from build123d import *

# Parameters (mm, degrees)
BOX002_W          = 50
BOX002_H          = 10
BOX002_DEPTH      = 3
CYLINDER001_R     = 3
CYLINDER001_DEPTH = 5
CYLINDER_R        = 10
CYLINDER_DEPTH    = 3
CYLINDER003_R     = 3
CYLINDER003_DEPTH = 5
CYLINDER002_R     = 10
CYLINDER002_DEPTH = 3
BOX001_W          = 36
BOX001_H          = 85
BOX001_DEPTH      = 15
BOX_W             = 23
BOX_H             = 15
BOX_DEPTH         = 13
SKETCH_W          = 40
SKETCH_H          = 90
PAD_DEPTH         = 16
SKETCH001_W       = 32
SKETCH001_H       = 83.75
POCKET_DEPTH      = 13


with BuildPart() as cube002:
    # Box002 → Box002 (new body)
    with BuildSketch(Plane(origin=(-25, -13, 9), x_dir=(1, 0, 0), z_dir=(0, 0, 1))):
        with Locations((25, 5)):
            Rectangle(BOX002_W, BOX002_H)
    extrude(amount=BOX002_DEPTH)


with BuildPart() as cylinder001:
    # Cylinder001 → Cylinder001 (new body)
    with BuildSketch(Plane(origin=(0, -48.5, -1), x_dir=(1, 0, 0), z_dir=(0, 0, 1))):
        Circle(CYLINDER001_R)
    extrude(amount=CYLINDER001_DEPTH)


with BuildPart() as also_ful:
    # Cylinder → Cylinder (new body)
    with BuildSketch(Plane(origin=(0, -45, 0), x_dir=(1, 0, 0), z_dir=(0, 0, 1))):
        Circle(CYLINDER_R)
    extrude(amount=CYLINDER_DEPTH)

    # Cut002: cut Cylinder001
    add(cylinder001.part, mode=Mode.SUBTRACT)


with BuildPart() as cylinder003:
    # Cylinder003 → Cylinder003 (new body)
    with BuildSketch(Plane(origin=(0, 48.5, -1), x_dir=(1, 0, 0), z_dir=(0, 0, 1))):
        Circle(CYLINDER003_R)
    extrude(amount=CYLINDER003_DEPTH)


with BuildPart() as obj1:
    # Cylinder002 → Cylinder002 (new body)
    with BuildSketch(Plane(origin=(0, 45, 0), x_dir=(1, 0, 0), z_dir=(0, 0, 1))):
        Circle(CYLINDER002_R)
    extrude(amount=CYLINDER002_DEPTH)

    # Cut003: cut Cylinder003
    add(cylinder003.part, mode=Mode.SUBTRACT)


with BuildPart() as cube001:
    # Box001 → Box001 (new body)
    with BuildSketch(Plane(origin=(-18, -42.5, 5), x_dir=(1, 0, 0), z_dir=(0, 0, 1))):
        with Locations((18, 42.5)):
            Rectangle(BOX001_W, BOX001_H)
    extrude(amount=BOX001_DEPTH)


with BuildPart() as cube:
    # Box → Box (new body)
    with BuildSketch(Plane(origin=(-15.35, -49.3, 3), x_dir=(1, 0, 0), z_dir=(0, 0, 1))):
        with Locations((11.5, 7.5)):
            Rectangle(BOX_W, BOX_H)
    extrude(amount=BOX_DEPTH)


with BuildPart() as also:
    # Sketch → Pad (new body)
    with BuildSketch(Plane.XY):
        Rectangle(SKETCH_W, SKETCH_H)
    extrude(amount=PAD_DEPTH)

    # Sketch001 (on Face6 of Pad) → Pocket (cut)
    with BuildSketch(Plane.XY.offset(16)):
        Rectangle(SKETCH001_W, SKETCH001_H)
    extrude(amount=-POCKET_DEPTH, mode=Mode.SUBTRACT)

    # Cut: cut Cube
    add(cube.part, mode=Mode.SUBTRACT)

    # Cut001: cut Cube001
    add(cube001.part, mode=Mode.SUBTRACT)

    # Fusion: union also ful, obj1
    add(also_ful.part)
    add(obj1.part)

    # Cut004: cut Cube002
    add(cube002.part, mode=Mode.SUBTRACT)


solid = also.part
Could you check a few things on this model? Use its own coordinates, in mm. A direction names the side the tool comes from. Give positions to 0.01 mm unless a question says otherwise; leave off trailing zeros. Order: outer loops, then holes, each group sorted by start corner. A loop starts at its lowest first (then second) coordinate and runs counter-clockwise, first axis right, second up.
1. Suppose I cut it at C-C (x = 6). List the corners of the cut face in (y, z) for me (3 decimals).
2. For faces 4 (the flat face through (-19, -8, 12)), 5 (the flat face through (-17, -45, 6)), 6 (the cylindrical face through (0, -55, 1)), 7 (the flat face through (18, -1, 10)), 8 (the flat face through (-20, -1, 8)), which set-ups out of +Z, -Z, +X, -X, +Y, -Y let a thin tool reach every point of the face, with its end or its side?
3. Suppose I cut it at D-D (y = -48.5). List the corners of the cut face in (x, z) for me.
4. Will these pins go through, and if not, where does the flat tip stop? P1, Ø4, axis at x = -6, z = 8, coming from the +Y side; P2, Ø1.5, axis at x = -10.5, y = 40, coming from the +Z side; P3, Ø1.6, axis at x = 3, z = 3.5, coming from the -Y side; P4, Ø5, axis at x = 0, y = 48.5, coming from the +Z side.
5. I need wall thicknesses on L1, parallel to Y at x = 0, z = 1.65; L2, parallel to X at y = -39, z = 13.75; L3, parallel to Y at x = 16, z = 7. Which ranges of each line are inside material? Lowest first, please.
6. We'd pull the mould along Z, two halves only. Please class faces 1 (the flat face through (19, 7, 16)), 2 (the flat face through (0, 42.5, 10)), 3 (the flat face through (19, -8, 12)): pulls with the +Z half, pulls with the -Z half, needs draft (parallel to the pull), parting line crosses it, or undercut.
7. Suppose I cut it at A-A (x = 0). List the corners of the cut face in (y, z) for me (3 decimals).
8. Suppose I cut it at B-B (z = 1). List the corners of the cut face in (x, y) for me.
Solved:
1. outline: (-53, 0) - (53, 0) - (53, 3) - (45, 3) - (45, 16) - (42.5, 16) - (42.5, 5) - (41.875, 5) - (41.875, 3) - (-53, 3) - close
2. face 4: +X, -X
2. face 5: +Z, -Z, -X, -Y
2. face 6: +Z, -Z, -Y
2. face 7: +Z
2. face 8: +Z, -Z, -X, +Y, -Y
3. outline: (-9.37, 0) - (-3, 0) - (-3, 3) - (-9.37, 3) - close; (3, 0) - (9.37, 0) - (9.37, 3) - (3, 3) - close
4. P1: stops at y = 45
4. P2: stops at z = 3
4. P3: stops at y = -54.71
4. P4: passes through
5. L1: y = -55 to -51.5, -45.5 to 45.5, 51.5 to 55
5. L2: x = -20 to -18, 18 to 20
5. L3: y = -45 to -42.5, 42.5 to 45
6. face 1: pulls with the +Z half
6. face 2: needs draft
6. face 3: undercut
7. outline: (-55, 0) - (-51.5, 0) - (-51.5, 3) - (-55, 3) - close; (-45.5, 0) - (45.5, 0) - (45.5, 3) - (45, 3) - (45, 16) - (42.5, 16) - (42.5, 5) - (41.875, 5) - (41.875, 3) - (-45.5, 3) - close; (51.5, 0) - (55, 0) - (55, 3) - (51.5, 3) - close
8. outline: (-20, -45) - (-10, -45) arc R10 ccw to (10, -45) - (20, -45) - (20, 45) - (10, 45) arc R10 ccw to (-10, 45) - (-20, 45) - close; hole circle Ø6 at (0, -48.5); hole circle Ø6 at (0, 48.5)
